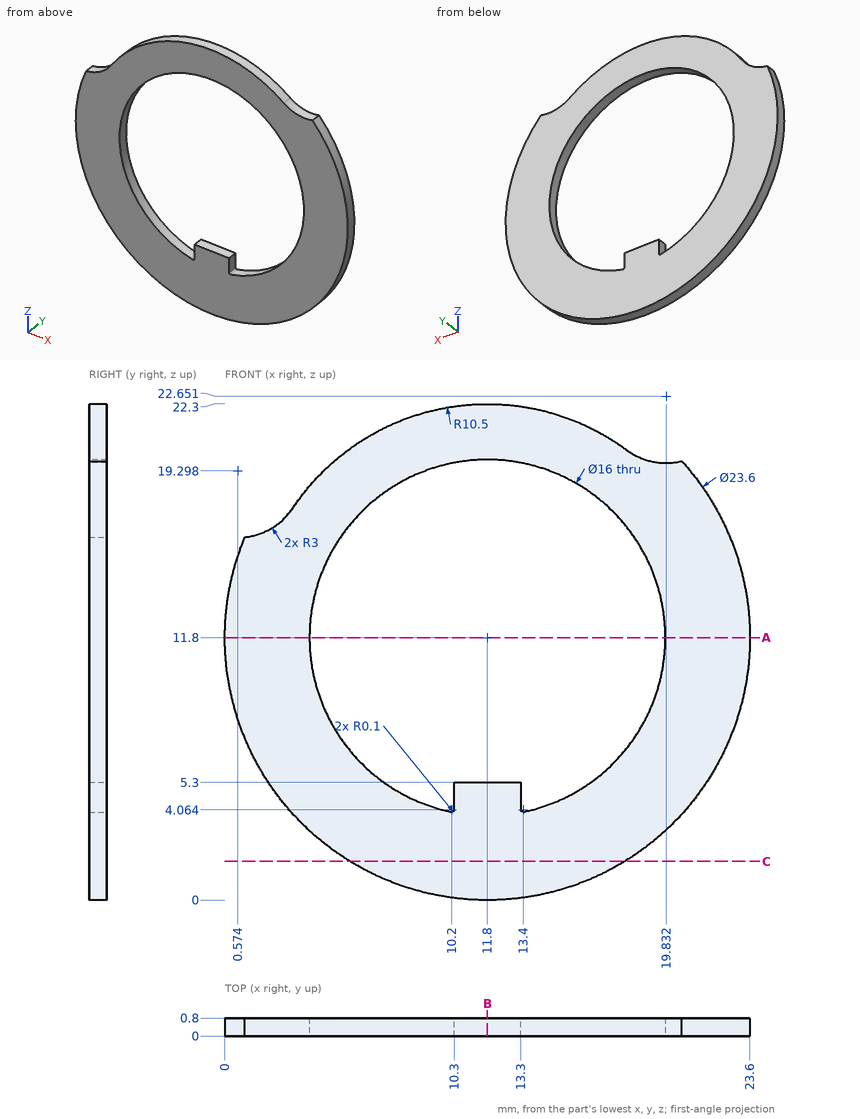
Here's the drawing with two shaded views (mm, measured from the low corner). I have some questions. Coordinates: 2 decimals unless noted, no trailing zeros. Order: outer loops, then holes, each group sorted by start corner. A loop starts at its lowest first (then second) coordinate and runs counter-clockwise, first axis right, second up. Notation, with made-up numbers: (8, 6) - (25, 6) arc R28 cw to (25, 38) - close; hole circle Ø11 at (81.25, 44). An arc over 180 degrees is marked (long way). Answer in a Markdown table with one row per item. Add a question column.
(1) I need wall thicknesses on L1, parallel to X at y = 0.55, z = 11.8; L2, parallel to X at y = 0.45, z = 6.25 (1 decimal); L3, parallel to Z at x = 15.5, y = 0.4 (1 decimal). Which ranges of each line are inside material? Lowest first, please.
(2) If we section it at A-A, the plane z = 11.8: Please give me the cut outline in (x, y).
(3) Will this pin go through, and if not, where does the flat tip stop? pin 1 (2 mm diameter, centred on x = 8, z = 16.5, fed in from +Y).
(4) If we section it at B-B, the plane x = 11.8: Please give me the cut outline in (y, z).
(5) If we section it at C-C, the plane z = 1.75: Please give me the cut outline in (x, y).
Results are:
| question | item | result |
|---|---|---|
| 1 | L1 | x = 0 to 3.8, 19.8 to 23.6 |
| 1 | L2 | x = 1.4 to 6, 17.6 to 22.2 |
| 1 | L3 | z = 0.6 to 4.7, 18.9 to 21.6 |
| 2 | outline | (0, 0) - (3.8, 0) - (3.8, 0.8) - (0, 0.8) - close; (19.8, 0) - (23.6, 0) - (23.6, 0.8) - (19.8, 0.8) - close |
| 3 | pin 1 | passes through |
| 4 | outline | (0, 0) - (0.8, 0) - (0.8, 5.3) - (0, 5.3) - close; (0, 19.8) - (0.8, 19.8) - (0.8, 22.3) - (0, 22.3) - close |
| 5 | outline | (5.62, 0) - (17.98, 0) - (17.98, 0.8) - (5.62, 0.8) - close |
